CAD build for the part. Positions are in the model's coordinates, mm. Face numbers are marked on the shaded views. A direction names the side the tool comes from. Give positions to 0.01 mm unless a question says otherwise; leave off trailing zeros. Write each loop counter-clockwise with the first axis right and the second up, starting at its lowest first coordinate (ties: lowest second). Pieces come first, ordered by that corner, then holes. Notation, with made-up numbers: (18, -2.5) - (73, -2.5) arc R20 ccw to (73, 23.5) - close; hole circle Ø4 at (-32, -23.75). An arc over 180 degrees is marked (long way). Write item = value, one per line. Start each with the question number.
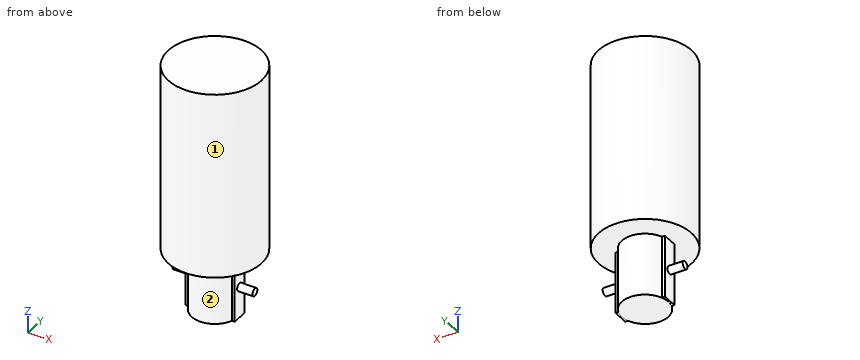
```python
from build123d import *

# Parameters (mm, degrees)
F0_R     = 15
F1_DEPTH = 60
F2_R     = 7.5
F3_DEPTH = 20
F6_DEPTH = 1
F7_R     = 1.25
F8_DEPTH = 5


with BuildPart() as f1:
    # F0 (on Top) → F1 (new body)
    with BuildSketch(Plane.XY):
        Circle(F0_R)
    extrude(amount=F1_DEPTH)

    # F2 (on Top) → F3 (join)
    with BuildSketch(Plane.XY):
        Circle(F2_R)
    extrude(amount=-F3_DEPTH)

    # F5 (on offset) → F6 (join)
    with BuildSketch(Plane.YZ.offset(7)):
        Polygon((-2.499352, 0), (-2.499352, -20), (2.499352, -19.886207), (2.499352, 0), align=None)
    extrude(amount=F6_DEPTH)

    # F7 (on face) → F8 (join)
    with BuildSketch(Plane.YZ.offset(8)):
        with Locations((0.000648, -9.943104)):
            Circle(F7_R)
    extrude(amount=F8_DEPTH)

    # F9: F1 across plane


with BuildPart() as f1_1:
    add(f1.part)
    add(f1.part.mirror(Plane.YZ))


solid = f1_1.part
```
1. Tool access for the marked faces 1 and 2: list every direction of +Z, -Z, +X, -X, +Y, -Y with a clear straight run to the whole face (end or side of a thin tool).
2. Wall check: line 1 along Z through (x, y) = (3.25, 8.5); line 2 along X through (y, z) = (-0.5, 3); line 3 along X through (y, z) = (-2.25, -4). Give the ranges that are in metal, low to high.
3. Cut at A-A (z = -7.5). Give the cut face in (x, y), then the cut area to 3 significant figures.
4. Cut at C-C (x = 9.25). Give the cut face in (y, z), then the cut area to 3 significant figures.
5. Cut at D-D (y = 0). Give the cut face in (x, z), then the cut area to 3 significant figures.
6. Pin check, flat tips, straight feed: pin 1 Ø0.5 at (x, z) = (7.5, -8) entering from -Y; pin 2 Ø12 at (x, z) = (5.5, 22.5) entering from -Y; pin 3 Ø6 at (y, z) = (5, -5) entering from +X; pin 4 Ø1.2 at (y, z) = (0.5, -9.5) entering from +X. Stop position of each tip, or through.
7. Cut at B-B (x = 0). Give the cut face in (y, z).
Output:
q1.face_1 = +Z, -Z
q1.face_2 = -Z, -Y
q2.line_1 = 0 to 60
q2.line_2 = -14.99 to 14.99
q2.line_3 = -8 to 8
q3.outline = (-8, -2.5) - (-7.07, -2.5) arc R7.5 ccw to (7.07, -2.5) - (8, -2.5) - (8, 2.5) - (7.07, 2.5) arc R7.5 ccw to (-7.07, 2.5) - (-8, 2.5) - close
q3.area = 183 mm2
q4.outline = (-11.81, 0) - (11.81, 0) - (11.81, 60) - (-11.81, 60) - close; circle Ø2.5 at (0, -9.94)
q4.area = 1,420 mm2
q5.outline = (-15, 0) - (-8, 0) - (-8, -8.69) - (-13, -8.69) - (-13, -11.19) - (-8, -11.19) - (-8, -19.94) - (-7.5, -19.94) - (-7.5, -20) - (7.5, -20) - (7.5, -19.94) - (8, -19.94) - (8, -11.19) - (13, -11.19) - (13, -8.69) - (8, -8.69) - (8, 0) - (15, 0) - (15, 60) - (-15, 60) - close
q5.area = 2,140 mm2
q6.pin_1 = -2.5
q6.pin_2 = -15
q6.pin_3 = 8
q6.pin_4 = 13
q7.outline = (-15, 0) - (-7.5, 0) - (-7.5, -20) - (7.5, -20) - (7.5, 0) - (15, 0) - (15, 60) - (-15, 60) - close
